from build123d import *

# Parameters (mm, degrees)
BOSS_EXTRUDE1_DEPTH                                 = 60
CBORE_FOR_M5_HEX_SOCKET_HEAD_CAP_SCREW1_D           = 5.3
CBORE_FOR_M5_HEX_SOCKET_HEAD_CAP_SCREW1_CBORE_D     = 10
CBORE_FOR_M5_HEX_SOCKET_HEAD_CAP_SCREW1_CBORE_DEPTH = 17.4
M6_CLEARANCE_HOLE1_D                                = 6.6
M6_CLEARANCE_HOLE1_DEPTH                            = 15
SKETCH8_W                                           = 20
SKETCH8_H                                           = 3
BOSS_EXTRUDE2_DEPTH                                 = 10
SKETCH9_W                                           = 60.5
SKETCH9_H                                           = 10
BOSS_EXTRUDE3_DEPTH                                 = 60
FILLET1_R                                           = 1
FILLET2_R                                           = 6
FILLET2_R_2                                         = 1
CHAMFER1_SIZE                                       = 0.6


with BuildPart() as part:
    # Sketch1 → Boss-Extrude1 (new body)
    with BuildSketch(Plane.XY):
        Polygon((30.25, 0), (-30.25, 0), (-30.25, 109), (-15.25, 109), (-15.25, 48), (15.25, 48), (15.25, 109), (30.25, 109), align=None)
    extrude(amount=BOSS_EXTRUDE1_DEPTH)

    # CBORE for M5 Hex Socket Head Cap Screw1 (through all)
    with Locations(Plane.XY.offset(60)):
        with Locations((-18, 7), (18, 7), (18, 39), (-18, 39)):
            CounterBoreHole(CBORE_FOR_M5_HEX_SOCKET_HEAD_CAP_SCREW1_D / 2, CBORE_FOR_M5_HEX_SOCKET_HEAD_CAP_SCREW1_CBORE_D / 2, CBORE_FOR_M5_HEX_SOCKET_HEAD_CAP_SCREW1_CBORE_DEPTH)

    # M6 Clearance Hole1
    with Locations(Plane.ZY.offset(30.25)):
        with Locations((48, 93), (13, 93), (13, 63), (48, 63)):
            m6_clearance_hole1 = Hole(M6_CLEARANCE_HOLE1_D / 2, depth=M6_CLEARANCE_HOLE1_DEPTH)

    # Mirror1: M6 Clearance Hole1 across plane
    add(m6_clearance_hole1.mirror(Plane(origin=(0, 0, 0), x_dir=(0, 0, 1), z_dir=(1, 0, 0))), mode=Mode.SUBTRACT)

    # Sketch8 → Boss-Extrude2 (add)
    with BuildSketch(Plane(origin=(0, 0, 0), x_dir=(-1, 0, 0), z_dir=(0, 0, -1))):
        with Locations((0, 46.5)):
            Rectangle(SKETCH8_W, SKETCH8_H)
    extrude(amount=BOSS_EXTRUDE2_DEPTH)

    # Sketch9 → Boss-Extrude3 (add)
    with BuildSketch(Plane.XY.offset(60)):
        with Locations((0, 114)):
            Rectangle(SKETCH9_W, SKETCH9_H)
    extrude(amount=-BOSS_EXTRUDE3_DEPTH)

    # Fillet1
    fillet1_edges = [part.edges().sort_by_distance(p)[0] for p in [
        (30.25, 119, 30),
        (-30.25, 119, 30),
        (-15.25, 48, 30),
        (15.25, 48, 30),
        (30.25, 0, 30),
        (-30.25, 0, 30),
    ]]
    fillet(fillet1_edges, radius=FILLET1_R)

    # Fillet2
    # the kernel refuses this fillet: 6, 1 mm, written as the material it adds along each edge
    with BuildSketch(Plane(origin=(10, 45, 0), x_dir=(1, 0, 0), z_dir=(0, 1, 0)), Plane(origin=(-10, 48, 0), x_dir=(-1, 0, 0), z_dir=(0, -1, 0))) as fillet2_piece_1:
        with BuildLine():
            CenterArc((FILLET2_R, FILLET2_R), FILLET2_R, 180, 90)
            Line((0, FILLET2_R), (0, 0))
            Line((0, 0), (FILLET2_R, 0))
        make_face()
    extrude(amount=3)
    # the kernel refuses this fillet: 6, 1 mm, written as the material it takes off along each edge
    with BuildSketch(Plane(origin=(10, 42.5, -10), x_dir=(-1, 0, 0), z_dir=(0, 1, 0))) as fillet2_2_piece_1:
        with BuildLine():
            CenterArc((FILLET2_R_2, FILLET2_R_2), FILLET2_R_2, 180, 90)
            Line((0, FILLET2_R_2), (0, 0))
            Line((0, 0), (FILLET2_R_2, 0))
        make_face()
    extrude(amount=8, mode=Mode.SUBTRACT)
    with BuildSketch(Plane(origin=(-10, 50.5, -10), x_dir=(0, 0, 1), z_dir=(0, -1, 0))) as fillet2_2_piece_2:
        with BuildLine():
            CenterArc((FILLET2_R_2, -FILLET2_R_2), FILLET2_R_2, 90, 90)
            Line((0, -FILLET2_R_2), (0, 0))
            Line((0, 0), (FILLET2_R_2, 0))
        make_face()
    extrude(amount=8, mode=Mode.SUBTRACT)

    # Chamfer1
    chamfer1_edges = [part.edges().sort_by_distance(p)[0] for p in [
        (0, 109, 60),
        (0, 119, 60),
        (-30.25, 59.5, 60),
        (0, 0, 60),
        (30.25, 59.5, 60),
        (-15.25, 79, 60),
        (0, 48, 60),
        (-29.957106781, 0.292893219, 60),
        (29.957106781, 0.292893219, 60),
        (29.957106781, 118.707106781, 60),
        (-29.957106781, 118.707106781, 60),
        (14.957106781, 48.292893219, 60),
        (-14.957106781, 48.292893219, 60),
        (15.25, 79, 60),
        (-23, 39, 60),
        (13, 39, 60),
        (13, 7, 60),
        (-23, 7, 60),
    ]]
    chamfer(chamfer1_edges, length=CHAMFER1_SIZE)


solid = part.part
Design review of the part built by this model. Coordinates are the model's own, in mm. A direction names the side the tool comes from. Round coordinates to 2 decimals unless told otherwise and drop trailing zeros. Order: outer loops, then holes, each group sorted by start corner. A loop starts at its lowest first (then second) coordinate and runs counter-clockwise, first axis right, second up.
1) Clearance check with flat-ended pins moving along their axes: pin 1 Ø4 at (y, z) = (93, 48) entering from -X; pin 2 Ø8.5 at (y, z) = (63, 48) entering from -X; pin 3 Ø1 at (x, y) = (-23, 64.5) entering from -Z; pin 4 Ø3.5 at (y, z) = (46.5, -7) entering from +X. State where each tip first meets the part, or that it passes through.
The answers:
pin 1: passes through
pin 2: stops at x = -30.25
pin 3: stops at z = 0
pin 4: stops at x = 10.05
2) Draft analysis for pull direction Y (two halves, no side actions). For faces 1 (the cylindrical face through (11.711, 46.479, -1.804)), 2 (the flat face through (-15.25, 79, 29)), 3 (the flat face through (0, 45, -5)), 4 (the flat face through (0, 119, 30)), state which applies: released by +Y, released by -Y, zero draft, split by the parting line, or undercut.
The answers:
face 1: zero draft
face 2: undercut
face 3: released by -Y
face 4: released by +Y
3) Consider section D-D (y = 63). State the section outline as (x, z) points, plus the area to 3 significant figures.
The answers:
outline: (-30.25, 0) - (-15.25, 0) - (-15.25, 9.7) - (-30.25, 9.7) - close; (-30.25, 16.3) - (-15.25, 16.3) - (-15.25, 44.7) - (-30.25, 44.7) - close; (-30.25, 51.3) - (-15.25, 51.3) - (-15.25, 59.4) - (-15.85, 60) - (-29.65, 60) - (-30.25, 59.4) - close; (15.25, 0) - (30.25, 0) - (30.25, 9.7) - (15.25, 9.7) - close; (15.25, 16.3) - (30.25, 16.3) - (30.25, 44.7) - (15.25, 44.7) - close; (15.25, 51.3) - (30.25, 51.3) - (30.25, 59.4) - (29.65, 60) - (15.85, 60) - (15.25, 59.4) - close
area: 1,400 mm2
4) Machinability: for faces 5 (the flat face through (15.25, 79, 29)), 6 (the cylindrical face through (-22.64, 65.23, 50.43)), 7 (the cylindrical face through (-18.651, 43.957, 51.118)), which of the approach directions +Z, -Z, +X, -X, +Y, -Y give a long, thin tool a straight path to every point of the face, cutting with its end or side? Answer none if there is none.
The answers:
face 5: +Z, -Z
face 6: +X, -X
face 7: +Z
5) Consider section A-A (z = 13). Count the separate pieces of the cut face and the enclosed holes in it, plus the area to 3 significant figures.
The answers:
separate pieces: 4
enclosed holes: 4
area: 4,850 mm2
6) Consider section B-B (y = 79.5). State the section outline as (x, z) points, plus the area to 3 significant figures.
The answers:
outline: (-30.25, 0) - (-15.25, 0) - (-15.25, 59.4) - (-15.85, 60) - (-29.65, 60) - (-30.25, 59.4) - close; (15.25, 0) - (30.25, 0) - (30.25, 59.4) - (29.65, 60) - (15.85, 60) - (15.25, 59.4) - close
area: 1,800 mm2
7) For L1, parallel to Y at x = 18, z = 13; L2, parallel to Y at x = 21.75, z = 13; L3, parallel to Z at x = 19, y = 63, list the stretches that pass through material, from the lowest coordinate up.
The answers:
L1: y = 0 to 4.35, 9.65 to 36.35, 41.65 to 59.7, 66.3 to 89.7, 96.3 to 119
L2: y = 0 to 59.7, 66.3 to 89.7, 96.3 to 119
L3: z = 0 to 9.7, 16.3 to 44.7, 51.3 to 60
